```python
from build123d import *

# Parameters (mm, degrees)
PAD009_DEPTH    = 2.8
FILLET004_R     = 0.4
POCKET014_DEPTH = 2.801
SKETCH028_R     = 8.5
POCKET017_DEPTH = 2.801


with BuildPart() as part:
    # Sketch009 (on Face6 of ShapeBinder008) → Pad009 (new body)
    with BuildSketch(Plane.XZ.offset(60.5)):
        with BuildLine():
            Line((37.8, 3.2), (37.8, 0.4))
            Line((37.8, 0.4), (23.8, 0.4))
            ThreePointArc((23.8, 0.4), (23.4, 0), (23.8, -0.4))
            Line((23.8, -0.4), (37.8, -0.4))
            Line((37.8, -0.4), (37.8, -33.8))
            Line((37.8, -33.8), (23.8, -33.8))
            ThreePointArc((23.8, -33.8), (23.4, -34.2), (23.8, -34.6))
            Line((23.8, -34.6), (37.8, -34.6))
            Line((37.8, -34.6), (37.8, -37.4))
            Line((37.8, -37.4), (35.8, -38.15))
            Line((35.8, -38.15), (35.8, -37.4))
            Line((35.8, -37.4), (33, -37.4))
            Line((33, -37.4), (33, -39.4))
            Line((33, -39.4), (25.535898, -37.4))
            Line((25.535898, -37.4), (-25.535898, -37.4))
            Line((-25.535898, -37.4), (-33, -39.4))
            Line((-33, -39.4), (-33, -37.4))
            Line((-33, -37.4), (-35.8, -37.4))
            Line((-35.8, -38.15), (-35.8, -37.4))
            Line((-37.8, -37.4), (-35.8, -38.15))
            Line((-37.8, -37.4), (-37.8, -34.6))
            Line((-37.8, -34.6), (-23.8, -34.6))
            ThreePointArc((-23.8, -34.6), (-23.4, -34.2), (-23.8, -33.8))
            Line((-23.8, -33.8), (-37.8, -33.8))
            Line((-37.8, -33.8), (-37.8, -0.4))
            Line((-37.8, -0.4), (-23.8, -0.4))
            ThreePointArc((-23.8, -0.4), (-23.4, 0), (-23.8, 0.4))
            Line((-23.8, 0.4), (-37.8, 0.4))
            Line((-37.8, 0.4), (-37.8, 3.2))
            Line((-37.8, 3.2), (-35.8, 3.95))
            Line((-35.8, 3.95), (-35.8, 3.2))
            Line((-35.8, 3.2), (-33, 3.2))
            Line((-33, 3.2), (-33, 5.2))
            Line((-33, 5.2), (-25.535898, 3.2))
            Line((-25.535898, 3.2), (25.535898, 3.2))
            Line((25.535898, 3.2), (33, 5.2))
            Line((33, 5.2), (33, 3.2))
            Line((33, 3.2), (35.8, 3.2))
            Line((35.8, 2.45), (35.8, 3.2))
            Line((37.8, 3.2), (35.8, 2.45))
        make_face()
    extrude(amount=-PAD009_DEPTH)

    # Fillet004
    fillet004_edges = [part.edges().sort_by_distance(p)[0] for p in [
        (33, -59.1, 5.2),
        (37.8, -59.1, 3.2),
        (37.8, -59.1, 0.4),
        (37.8, -59.1, -0.4),
        (37.8, -59.1, -33.8),
        (37.8, -59.1, -34.6),
        (37.8, -59.1, -37.4),
        (33, -59.1, -39.4),
        (-37.8, -59.1, -33.8),
        (-37.8, -59.1, -34.6),
        (-37.8, -59.1, -37.4),
        (-33, -59.1, -39.4),
        (-33, -59.1, 5.2),
        (-37.8, -59.1, 3.2),
        (-37.8, -59.1, 0.4),
        (-37.8, -59.1, -0.4),
    ]]
    fillet(fillet004_edges, radius=FILLET004_R)

    # Sketch025 (on Face2 of Fillet004) → Pocket014 (cut, through all)
    with BuildSketch(Plane.XZ.offset(60.5)):
        with BuildLine():
            ThreePointArc((-24, -4.49), (-24.755, -5.245), (-24, -6))
            Line((-24, -6), (-12, -6))
            ThreePointArc((-12, -6), (-11.245, -5.245), (-12, -4.49))
            Line((-24, -4.49), (-12, -4.49))
        make_face()
        with BuildLine():
            ThreePointArc((12, -4.49), (11.245, -5.245), (12, -6))
            Line((12, -6), (24, -6))
            ThreePointArc((24, -6), (24.755, -5.245), (24, -4.49))
            Line((12, -4.49), (24, -4.49))
        make_face()
    extrude(amount=-POCKET014_DEPTH, mode=Mode.SUBTRACT)

    # Sketch028 (on Face2 of Pocket014) → Pocket017 (cut, through all)
    with BuildSketch(Plane.XZ.offset(60.5)):
        with Locations((-12.8, -24.1)):
            Circle(SKETCH028_R)
        with Locations((12.8, -24.1)):
            Circle(SKETCH028_R)
        with BuildLine():
            ThreePointArc((-2.85, -29.7), (-5.35, -32.2), (-2.85, -34.7))
            Line((-2.85, -34.7), (2.85, -34.7))
            ThreePointArc((2.85, -34.7), (5.35, -32.2), (2.85, -29.7))
            Line((-2.85, -29.7), (2.85, -29.7))
        make_face()
    extrude(amount=-POCKET017_DEPTH, mode=Mode.SUBTRACT)


solid = part.part
```
The listing builds one solid part. Answer for the finished solid, in the listing's coordinates (mm). A direction names the side the tool comes from. Coordinates: 2 decimals unless noted, no trailing zeros. Write each loop counter-clockwise with the first axis right and the second up, starting at its lowest first coordinate (ties: lowest second). Pieces come first, ordered by that corner, then holes. Notation, with made-up numbers: (48.5, 22.5) -> (87.5, 22.5) arc R26 ccw to (87.5, 50.5) -> close; hole circle Ø6 at (-34, 15.25). An arc over 180 degrees is marked (long way). Write each question's results on one line, items separated by ' | '. Start each with the question number.
1) A cutting plane is placed at C-C (y = -59.7). Count the separate pieces of the cut face and the enclosed holes in it, then the cut area to 3 significant figures.
2) A cutting plane is placed at D-D (z = -25.5). Determine the outline of the cut face in (x, y), then the cut area to 3 significant figures.
3) A cutting plane is placed at A-A (x = -12.8). Determine the outline of the cut face in (y, z), then the cut area to 3 significant figures.
4) A cutting plane is placed at B-B (x = 2). Determine the outline of the cut face in (y, z).
5) A tool of negligible diameter and unlimited length cuts with its end or side. For faces 4 (the flat face through (31, -59, -33.8)), 5 (the cylindrical face through (-24.755, -59.12, -5.228)), 6 (the flat face through (28.97, -59.12, 4.12)), from which of +Z, -Z, +X, -X, +Y, -Y can it reach the whole face along a straight path? Write none if from no direction.
6) For a pull along X with two mould halves and no side action, classify faces 1 (the flat face through (33, -59, 4)), 2 (the cylindrical face through (-5.35, -59.12, -32.15)), 3 (the flat face through (31, -59, 0.4)) as +X half, -X half, draft (parallel to the pull), parting line (faces both ways), or undercut.
7) Flat-ended cylindrical pins translate along their axes: pin 1 Ø1.6 at (y, z) = (-59.5, -38) entering from +X; pin 2 Ø0.8 at (x, y) = (7, -59.5) entering from -Z; pin 3 Ø1.2 at (y, z) = (-59, 4) entering from +X. Find the tip coordinate at first contact, or state that the pin passes through.
8) Straight lines are drawn through the part: probe 1 along Z at (x, y) = (12.8, -59.55); probe 2 along Z at (x, y) = (-27, -58.9); probe 3 along Z at (x, y) = (8, -59.6). For each, find the intervals that lie inside material, in ascending order.
Values follow:
1) separate pieces: 1 | enclosed holes: 5 | area: 2,510 mm²
2) outline: (-37.8, -60.5) -> (-21.18, -60.5) -> (-21.18, -57.7) -> (-37.8, -57.7) -> close; (-4.42, -60.5) -> (4.42, -60.5) -> (4.42, -57.7) -> (-4.42, -57.7) -> close; (21.18, -60.5) -> (37.8, -60.5) -> (37.8, -57.7) -> (21.18, -57.7) -> close | area: 118 mm²
3) outline: (-60.5, -37.4) -> (-57.7, -37.4) -> (-57.7, -32.6) -> (-60.5, -32.6) -> close; (-60.5, -15.6) -> (-57.7, -15.6) -> (-57.7, -6) -> (-60.5, -6) -> close; (-60.5, -4.49) -> (-57.7, -4.49) -> (-57.7, 3.2) -> (-60.5, 3.2) -> close | area: 61.9 mm²
4) outline: (-60.5, -37.4) -> (-57.7, -37.4) -> (-57.7, -34.7) -> (-60.5, -34.7) -> close; (-60.5, -29.7) -> (-57.7, -29.7) -> (-57.7, 3.2) -> (-60.5, 3.2) -> close
5) face 4: +X, +Y, -Y | face 5: +Y, -Y | face 6: +Z, +Y, -Y
6) face 1: +X half | face 2: undercut | face 3: draft
7) pin 1: x = 37.79 | pin 2: z = -37.4 | pin 3: x = 33
8) probe 1: -37.4 to -32.6, -15.6 to -6, -4.49 to 3.2 | probe 2: -37.79 to -34.6, -33.8 to -0.4, 0.4 to 3.59 | probe 3: -37.4 to -31.11, -17.09 to 3.2
